Model file for the job. Use its own axes, mm. A direction names the side the tool comes from. Give positions to 0.01 mm unless a question says otherwise; leave off trailing zeros. Write each loop counter-clockwise with the first axis right and the second up, starting at its lowest first coordinate (ties: lowest second). Pieces come first, ordered by that corner, then holes. Notation, with made-up numbers: (65, 70) - (79, 70) arc R24 ccw to (79, 91) - close; hole circle Ø4 at (-0.5, 22). An arc over 180 degrees is marked (long way). Use CSV: the item, a comma, the result in double quotes.
from build123d import *

# Parameters (mm, degrees)
SKETCH1_R           = 15
BOSS_EXTRUDE1_DEPTH = 2.5
CUT_EXTRUDE3_DEPTH  = 0.25
SKETCH3_R           = 2
CUT_EXTRUDE4_DEPTH  = 3.5


with BuildPart() as part:
    # Sketch1 → Boss-Extrude1 (new body)
    with BuildSketch(Plane(origin=(0, 0, 0), x_dir=(1, 0, 0), z_dir=(0, 1, 0))):
        Circle(SKETCH1_R)
    extrude(amount=BOSS_EXTRUDE1_DEPTH)

    # Sketch2 → Cut-Extrude3 (cut)
    with BuildSketch(Plane(origin=(0, 0, 0), x_dir=(1, 0, 0), z_dir=(0, 1, 0))):
        with BuildLine():
            Line((0, 0.850650808), (-8.412270287, 12.429147542))
            ThreePointArc((-8.412270287, 12.429147542), (-8.821675635, 12.141994852), (-9.221287282, 11.841362289))
            Line((-9.221287282, 11.841362289), (-0.809016994, 0.262865556))
            Line((-0.809016994, 0.262865556), (-14.420356242, -4.159726657))
            ThreePointArc((-14.420356242, -4.159726657), (-14.273771015, -4.637829342), (-14.111339247, -5.110783174))
            Line((-14.111339247, -5.110783174), (-0.5, -0.68819096))
            Line((-0.5, -0.68819096), (-0.5, -15))
            ThreePointArc((-0.5, -15), (0, -15.00833102), (0.5, -15))
            Line((0.5, -15), (0.5, -0.68819096))
            Line((0.5, -0.68819096), (14.111339247, -5.110783174))
            ThreePointArc((14.111339247, -5.110783174), (14.273771015, -4.637829342), (14.420356242, -4.159726657))
            Line((14.420356242, -4.159726657), (0.809016994, 0.262865556))
            Line((0.809016994, 0.262865556), (9.221287282, 11.841362289))
            ThreePointArc((9.221287282, 11.841362289), (8.821675635, 12.141994852), (8.412270287, 12.429147542))
            Line((8.412270287, 12.429147542), (0, 0.850650808))
        make_face()
    extrude(amount=CUT_EXTRUDE3_DEPTH, mode=Mode.SUBTRACT)

    # Sketch3 → Cut-Extrude4 (cut, through all)
    with BuildSketch(Plane(origin=(0, 0, 0), x_dir=(1, 0, 0), z_dir=(0, 1, 0))):
        Circle(SKETCH3_R)
    extrude(amount=CUT_EXTRUDE4_DEPTH, mode=Mode.SUBTRACT)


solid = part.part
(1) Pull direction X, two halves, no side cores. Call faces 3 (the face through (0, 0.25, 8)), 4 (the face through (-14.985, 1.232, -0.66)), 5 (the face through (6, 0, 8)): released by +X, released by -X, zero draft, split by the parting line, or undercut.
Checked values:
face 3,"undercut"
face 4,"split by the parting line"
face 5,"zero draft"
(2) 3-axis set-ups, long thin cutter, end or side, ignore diameter. For faces 1 (the face through (-5, 0.25, -7)), 2 (the face through (-6, 0, 8)): which of +Z, -Z, +X, -X, +Y, -Y reach the whole face in a straight line?
Checked values:
face 1,"-Y"
face 2,"+Z, -Z, +X, -X, -Y"
(3) Saw through at A-A, the plane x = 0. List the corners of the cut face in (y, z).
Checked values:
outline,"(0, -15) - (2.5, -15) - (2.5, -2) - (0, -2) - close; (0.25, 2) - (2.5, 2) - (2.5, 15) - (0.25, 15) - close"
(4) Saw through at D-D, the plane x = 5. List the corners of the cut face in (y, z).
Checked values:
outline,"(0, -14.14) - (2.5, -14.14) - (2.5, 14.14) - (0, 14.14) - (0, 2.15) - (0.25, 2.15) - (0.25, 1.1) - (0, 1.1) - (0, -6.03) - (0.25, -6.03) - (0.25, -7.73) - (0, -7.73) - close"
(5) Saw through at B-B, the plane y = 1. List the corners of the cut face in (x, z), then the cut area to 3 significant figures.
Checked values:
outline,"circle Ø30 at (0, 0); hole circle Ø4 at (0, 0)"
area,"694 mm^2"
(6) Wall check: probe 1 along X at (y, z) = (1.7, 0); probe 2 along Z at (x, y) = (12.25, 0.2). Give the ranges that are in metal, low to high. Write a range as [from, to].
Checked values:
probe 1,"x = [-15, -2], [2, 15]"
probe 2,"z = [-8.66, 3.45], [4.51, 8.66]"
(7) Saw through at C-C, the plane z = -10. List the corners of the cut face in (x, y).
Checked values:
outline,"(-11.18, 0) - (-7.88, 0) - (-7.88, 0.25) - (-6.65, 0.25) - (-6.65, 0) - (6.65, 0) - (6.65, 0.25) - (7.88, 0.25) - (7.88, 0) - (11.18, 0) - (11.18, 2.5) - (-11.18, 2.5) - close"
(8) Flat gauge pins, fed straight in: P1, Ø1, axis at x = -5.5, y = 1.5, coming from the -Z side; P2, Ø1, axis at x = 5.5, y = 0.5, coming from the +Z side; P3, Ø1.5, axis at x = -7, y = 2, coming from the +Z side. Where does each tip first touch, or does it go through?
Checked values:
P1,"stops at z = -14.14"
P2,"stops at z = 14.14"
P3,"stops at z = 13.64"
